Job drawing, mm, ordinate dimensions from the low corner. One solid piece. A direction names the side the tool comes from. Coordinates: 2 decimals unless noted, no trailing zeros. Order: outer loops, then holes, each group sorted by start corner. A loop starts at its lowest first (then second) coordinate and runs counter-clockwise, first axis right, second up. Notation, with made-up numbers: (-13, 36.5) - (17, 36.5) arc R24 ccw to (17, 64.5) - close; hole circle Ø10 at (54.5, -21). An arc over 180 degrees is marked (long way). Return JSON: item names as keys, results as strings.
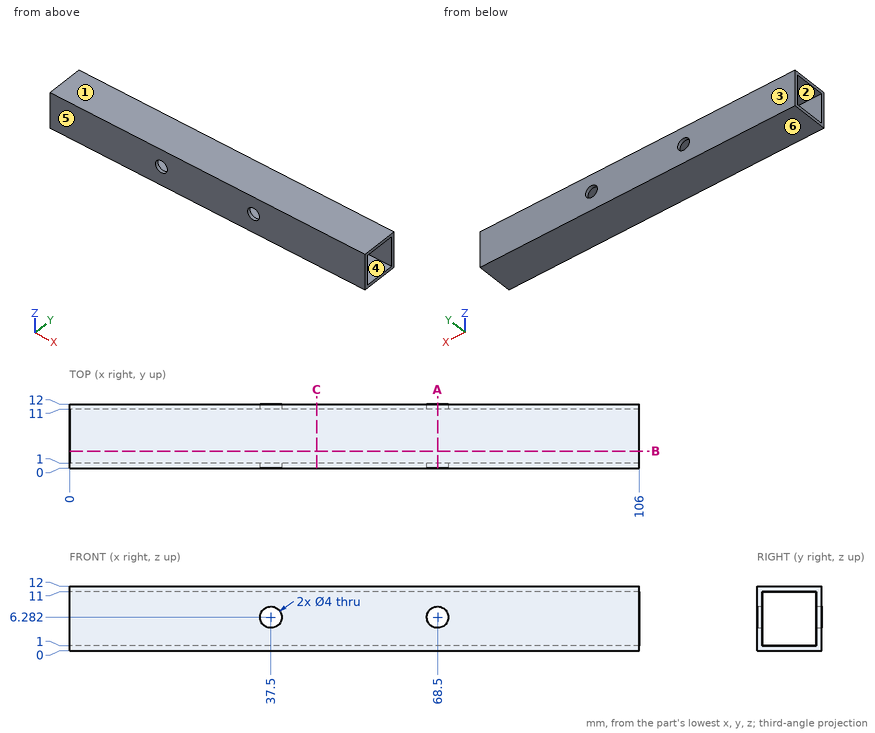
1. Drop flat-ended pins along their axis: pin 1 (3 mm diameter, centred on x = 68.5, z = 6.28, fed in from +Y); pin 2 (4 mm diameter, centred on y = 10.5, z = 1.5, fed in from +X). Give the stop position or say it passes through.
Check values:
{"pin 1": "through", "pin 2": "x = 106"}
2. Cut at A-A on x = 68.5. Give the cut face in (y, z), plus the area to 3 significant figures.
Check values:
{"outline": "(0, 0) - (12, 0) - (12, 4.28) - (11, 4.28) - (11, 1) - (1, 1) - (1, 4.28) - (0, 4.28) - close; (0, 8.28) - (1, 8.28) - (1, 11) - (11, 11) - (11, 8.28) - (12, 8.28) - (12, 12) - (0, 12) - close", "area": "36.0 mm²"}
3. Cut at B-B on y = 3.25. Give the cut face in (x, z), plus the area to 3 significant figures.
Check values:
{"outline": "(0, 0) - (106, 0) - (106, 1) - (0, 1) - close; (0, 11) - (106, 11) - (106, 12) - (0, 12) - close", "area": "212 mm²"}
4. Cut at C-C on x = 46. Give the cut face in (y, z).
Check values:
{"outline": "(0, 0) - (12, 0) - (12, 12) - (0, 12) - close; hole (1, 1) - (11, 1) - (11, 11) - (1, 11) - close"}
5. Mould opens along Y. For the marked faces 3, 4, 5 and 6 say: pulls with the +Y half, pulls with the -Y half, needs draft (parallel to the pull), parting line crosses it, or undercut.
Check values:
{"face 3": "pulls with the +Y half", "face 4": "undercut", "face 5": "pulls with the -Y half", "face 6": "needs draft"}
6. Tool access for the marked faces 1 and 2: list every direction of +Z, -Z, +X, -X, +Y, -Y with a clear straight run to the whole face (end or side of a thin tool).
Check values:
{"face 1": "+Z, +X, -X, +Y, -Y", "face 2": "+X, -X"}
7. Probe L1, parallel to X at y = 0.5, z = 6; L2, parallel to Y at x = 78, z = 2.5. List the from-to ranges inside material, lowest first.
Check values:
{"L1": "0 to 35.52, 39.48 to 66.52, 70.48 to 106", "L2": "0 to 1, 11 to 12"}
